The listing builds one solid part. Answer for the finished solid, in the listing's coordinates (mm). A direction names the side the tool comes from. Give positions to 0.01 mm unless a question says otherwise; leave off trailing zeros. Loops run counter-clockwise (first coordinate to the right, second up) from the corner with the lowest first, then second, coordinate; pieces in that order, holes last. Notation, with made-up numbers: (-17, 63.25) - (18, 63.25) arc R24 cw to (18, 94.25) - close; hole circle Ø11 at (15.25, -37.5). An arc over 180 degrees is marked (long way). Answer in a Markdown table with one row per item. Add a question column.
```python
from build123d import *

# Parameters (mm, degrees)
SKETCH_1_R               = 11
SKETCH_1_R_2             = 1.5
SKETCH_1_R_3             = 2.5
EXTRUDE_1_DEPTH          = 2
SKETCH_2_R               = 5
SKETCH_2_R_2             = 2.5
EXTRUDE_2_DEPTH          = 10
CUT_EXTRUDE_1_DEPTH      = 20.646882704
CUT_EXTRUDE_1_DEPTH_BACK = 20.646882704
SKETCH_3_R               = 1.5


with BuildPart() as part:
    # Эскиз1 → Бобышка-Вытянуть1 (new body)
    with BuildSketch(Plane.XY):
        Circle(SKETCH_1_R)
        with Locations((-8, 0)):
            Circle(SKETCH_1_R_2, mode=Mode.SUBTRACT)
        with Locations((0, 8)):
            Circle(SKETCH_1_R_2, mode=Mode.SUBTRACT)
        with Locations((8, 0)):
            Circle(SKETCH_1_R_2, mode=Mode.SUBTRACT)
        with Locations((0, -8)):
            Circle(SKETCH_1_R_2, mode=Mode.SUBTRACT)
        Circle(SKETCH_1_R_3, mode=Mode.SUBTRACT)
    extrude(amount=EXTRUDE_1_DEPTH)

    # Эскиз2 → Бобышка-Вытянуть2 (add)
    with BuildSketch(Plane.XY.offset(2)):
        Circle(SKETCH_2_R)
        Circle(SKETCH_2_R_2, mode=Mode.SUBTRACT)
    extrude(amount=EXTRUDE_2_DEPTH)

    # Эскиз3 → Вырез-Вытянуть1 (cut, two sides: drawn at the far end of the back side and taken through both)
    with BuildSketch(Plane(origin=(0, 0, 0), x_dir=(1, 0, 0), z_dir=(0, 1, 0)).offset(-CUT_EXTRUDE_1_DEPTH_BACK)):
        with Locations(Location((0, -7, 0), (0, 0, 270))):
            Circle(SKETCH_3_R)
    extrude(amount=CUT_EXTRUDE_1_DEPTH + CUT_EXTRUDE_1_DEPTH_BACK, mode=Mode.SUBTRACT)


solid = part.part
```
(1) A cutting plane is placed at C-C on x = 0. Determine the outline of the cut face in (y, z).
(2) A cutting plane is placed at D-D on y = -3.5. Determine the outline of the cut face in (x, z), plus the area to 3 significant figures.
(3) A cutting plane is placed at B-B on x = -9. Determine the outline of the cut face in (y, z).
(4) A cutting plane is placed at A-A on y = 0. Determine the outline of the cut face in (x, z).
(5) A tool of negligible diameter and unlimited length cuts with its end or side. For faces 1 (the face through (5, -2, 2)), 2 (the face through (0, 3, 0)), from which of +Z, -Z, +X, -X, +Y, -Y can it reach the whole face along a straight path? Write none if from no direction.
(6) Find the intervals of material crossed by line 1 along Y through (x, z) = (0, 0.75); line 2 along X through (y, z) = (-1.5, 8.25); line 3 along X through (y, z) = (0.5, 0.75), in increasing order. Write a range as [from, to].
(7) The mould has two halves that part along Y. Classify faces 3 (the face through (-2.38, -10.74, 0.99)), 4 (the face through (-0.575, 3.482, 8.386)), 5 (the face through (-9.5, 0.07, 0.99)): pulls with the +Y half, pulls with the -Y half, needs draft (parallel to the pull), parting line crosses it, or undercut.
(8) Given pin 1 Ø4 at (x, z) = (-5, 5) entering from -Y; pin 2 Ø1.5 at (x, y) = (-4, -8) entering from +Z; pin 3 Ø6 at (x, z) = (8, 3.5) entering from +Y, each flat-ended and moving along its own axis, determine where each tip first touches the part or whether it passes through.
Evaluation:
| question | item | result |
|---|---|---|
| 1 | outline | (-11, 0) - (-9.5, 0) - (-9.5, 2) - (-11, 2) - close; (-6.5, 0) - (-2.5, 0) - (-2.5, 5.5) - (-5, 5.5) - (-5, 2) - (-6.5, 2) - close; (-5, 8.5) - (-2.5, 8.5) - (-2.5, 12) - (-5, 12) - close; (2.5, 0) - (6.5, 0) - (6.5, 2) - (5, 2) - (5, 5.5) - (2.5, 5.5) - close; (2.5, 8.5) - (5, 8.5) - (5, 12) - (2.5, 12) - close; (9.5, 0) - (11, 0) - (11, 2) - (9.5, 2) - close |
| 2 | outline | (-10.43, 0) - (10.43, 0) - (10.43, 2) - (3.57, 2) - (3.57, 12) - (-3.57, 12) - (-3.57, 2) - (-10.43, 2) - close; hole circle Ø3 at (0, 7) |
| 2 | area | 106 mm² |
| 3 | outline | (-6.32, 0) - (-1.12, 0) - (-1.12, 2) - (-6.32, 2) - close; (1.12, 0) - (6.32, 0) - (6.32, 2) - (1.12, 2) - close |
| 4 | outline | (-11, 0) - (-9.5, 0) - (-9.5, 2) - (-11, 2) - close; (-6.5, 0) - (-2.5, 0) - (-2.5, 12) - (-5, 12) - (-5, 2) - (-6.5, 2) - close; (2.5, 0) - (6.5, 0) - (6.5, 2) - (5, 2) - (5, 12) - (2.5, 12) - close; (9.5, 0) - (11, 0) - (11, 2) - (9.5, 2) - close |
| 5 | face 1 | +Z |
| 5 | face 2 | -Z, +X, -X, +Y, -Y |
| 6 | line 1 | y = [-11, -9.5], [-6.5, -2.5], [2.5, 6.5], [9.5, 11] |
| 6 | line 2 | x = [-4.77, -2], [2, 4.77] |
| 6 | line 3 | x = [-10.99, -9.41], [-6.59, -2.45], [2.45, 6.59], [9.41, 10.99] |
| 7 | face 3 | parting line crosses it |
| 7 | face 4 | needs draft |
| 7 | face 5 | undercut |
| 8 | pin 1 | stops at y = -4 |
| 8 | pin 2 | stops at z = 2 |
| 8 | pin 3 | stops at y = 9.58 |
